The model under review builds one solid part; all positions refer to its coordinate system, in mm. A direction names the side the tool comes from. Coordinates: 2 decimals unless noted, no trailing zeros. Write each loop counter-clockwise with the first axis right and the second up, starting at its lowest first coordinate (ties: lowest second). Pieces come first, ordered by that corner, then holes. Notation, with made-up numbers: (-25, 71) - (-13, 71) arc R25 ccw to (-13, 91) - close; hole circle Ø8 at (18.25, -3). An arc over 180 degrees is marked (long way). Return JSON: item names as keys, results as strings. Group by question number.
(1) For pin 1 Ø10 at (x, y) = (6, 2.5) entering from +Z; pin 2 Ø5 at (x, y) = (33, 2) entering from -Z; pin 3 Ø2 at (y, z) = (-4.5, 1.5) entering from +X, all flat-tipped, find the tip position at first contact; note any pin that passes through.
(2) Draft analysis for pull direction X (two halves, no side actions). For faces 1 (the face through (63.787, 12.847, 1.972)), 2 (the face through (6, -27, 2)), 3 (the face through (61.526, 21.481, 1.972)), 4 (the face through (-14.677, 8.918, 2.028)), state which applies: released by +X, released by -X, zero draft, split by the parting line, or undercut.
(3) Tool access review of faces 5 (the face through (23.843, 19.422, 2.028)), 6 (the face through (24, 27, 2)): name each direction out of +Z, -Z, +X, -X, +Y, -Y from which nothing blocks a thin tool from reaching the whole face with its end or side.
(4) We need section A-A on x = 14.95. State the section outline as (y, z) points.
(5) To check wall thickness, follow L1, parallel to Y at x = 14.95, z = 1.05; L2, parallel to Y at x = 35, z = 2.55; L3, parallel to X at y = -10, z = 0.35. State the ranges of each line that lie inside material, in increasing order. Write a range as from..to.
(6) We need section C-C on y = 2. State the section outline as (x, z) points, then the cut area to 3 significant figures.
(7) We need section D-D on y = 11. State the section outline as (x, z) points.
(8) We need section B-B on z = 0.9. Give the number of separate pieces and of enclosed holes in the cut face, then the cut area to 3 significant figures.
```python
from build123d import *

# Parameters (mm, degrees)
SKETCH_1_R          = 3.1
SKETCH_1_R_2        = 1.6
SKETCH_1_W          = 20.4
SKETCH_1_H          = 40.4
EXTRUDE_1_DEPTH     = 4
FILLET_1_R          = 0.2
SKETCH_2_R          = 2.1
CUT_EXTRUDE_1_DEPTH = 4
CUT_EXTRUDE_2_DEPTH = 10


with BuildPart() as part:
    # 草图1 → 凸台-拉伸1 (new body)
    with BuildSketch(Plane.XY):
        with BuildLine():
            Line((-10.2, 27), (60.15625, 27))
            ThreePointArc((60.15625, 27), (63.954895943, 25.251198086), (65.096310169, 21.228115599))
            Line((65.096310169, 21.228115599), (62.440060169, 4.228115599))
            ThreePointArc((62.440060169, 4.228115599), (61.816569536, 2.476663431), (60.596300169, 1.074070141))
            Line((60.596300169, 1.074070141), (27.72371786, -24.851859719))
            ThreePointArc((27.72371786, -24.851859719), (24.808418455, -26.447713935), (21.531117522, -27))
            Line((21.531117522, -27), (-10.2, -27))
            ThreePointArc((-10.2, -27), (-17.271067812, -24.071067812), (-20.2, -17))
            Line((-20.2, -17), (-20.2, 17))
            ThreePointArc((-20.2, 17), (-17.271067812, 24.071067812), (-10.2, 27))
        make_face()
        with Locations((33, 2)):
            Circle(SKETCH_1_R, mode=Mode.SUBTRACT)
        with Locations((60, 21)):
            Circle(SKETCH_1_R_2, mode=Mode.SUBTRACT)
        with Locations((57.5, 5)):
            Circle(SKETCH_1_R_2, mode=Mode.SUBTRACT)
        Rectangle(SKETCH_1_W, SKETCH_1_H, mode=Mode.SUBTRACT)
    extrude(amount=EXTRUDE_1_DEPTH)

    # 圆角1
    fillet_1_edges = [part.edges().sort_by_distance(p)[0] for p in [
        (-10.2, 20.2, 2),
        (-10.2, -20.2, 2),
        (10.2, -20.2, 2),
        (10.2, 20.2, 2),
    ]]
    fillet(fillet_1_edges, radius=FILLET_1_R)

    # 草图2 → 切除-拉伸1 (cut)
    with BuildSketch(Plane.XY.offset(4)):
        with Locations((14.95, 11)):
            Circle(SKETCH_2_R)
        with Locations(Location((14.95, -11, 0), (0, 0, 180))):
            Circle(SKETCH_2_R)
        with Locations((-14.95, -11)):
            Circle(SKETCH_2_R)
        with Locations(Location((-14.95, 11, 0), (0, 0, 180))):
            Circle(SKETCH_2_R)
    extrude(amount=-CUT_EXTRUDE_1_DEPTH, mode=Mode.SUBTRACT)

    # 草图3 → 切除-拉伸2 (cut)
    with BuildSketch(Plane.XY.offset(4)):
        with BuildLine():
            Line((25.798016292, 21), (51.43418263, 21))
            ThreePointArc((51.43418263, 21), (53.713370196, 19.950718852), (54.398218731, 17.536869359))
            Line((54.398218731, 17.536869359), (52.852232934, 7.642560256))
            ThreePointArc((52.852232934, 7.642560256), (51.264559821, 5.440053089), (48.549531682, 5.420923567))
            Line((48.549531682, 5.420923567), (24.905572858, 17.210155114))
            ThreePointArc((24.905572858, 17.210155114), (23.851263897, 19.458426781), (25.798016292, 21))
        make_face()
    extrude(amount=-CUT_EXTRUDE_2_DEPTH, mode=Mode.SUBTRACT)


solid = part.part
```
Ans:
{
 "1": {"pin 1": "z = 4", "pin 2": "through", "pin 3": "x = 54.8"},
 "2": {"face 1": "released by +X", "face 2": "zero draft", "face 3": "undercut", "face 4": "undercut"},
 "3": {"face 5": "+Z, -Z", "face 6": "+Z, -Z, +X, -X, +Y"},
 "4": {"outline": "(-27, 0) - (-13.1, 0) - (-13.1, 4) - (-27, 4) - close; (-8.9, 0) - (8.9, 0) - (8.9, 4) - (-8.9, 4) - close; (13.1, 0) - (27, 0) - (27, 4) - (13.1, 4) - close"},
 "5": {"L1": "-27..-13.1, -8.9..8.9, 13.1..27", "L2": "-19.11..-0.37, 4.37..12.18, 21..27", "L3": "-20.2..-16.8, -13.1..-10.2, 10.2..13.1, 16.8..46.56"},
 "6": {"outline": "(-20.2, 0) - (-10.2, 0) - (-10.2, 4) - (-20.2, 4) - close; (10.2, 0) - (29.9, 0) - (29.9, 4) - (10.2, 4) - close; (36.1, 0) - (61.5, 0) - (61.5, 4) - (36.1, 4) - close", "area": "220 mm²"},
 "7": {"outline": "(-20.2, 0) - (-17.05, 0) - (-17.05, 4) - (-20.2, 4) - close; (-12.85, 0) - (-10.2, 0) - (-10.2, 4) - (-12.85, 4) - close; (10.2, 0) - (12.85, 0) - (12.85, 4) - (10.2, 4) - close; (17.05, 0) - (37.36, 0) - (37.36, 4) - (17.05, 4) - close; (53.38, 0) - (63.5, 0) - (63.5, 4) - (53.38, 4) - close"},
 "8": {"separate pieces": "1", "enclosed holes": "9", "area": "2,660 mm²"}
}
